Input: part model. Units: mm. Frame: model coordinates. A direction names the side the tool comes from. Give positions to 0.01 mm unless a question says otherwise; leave off trailing zeros. Order: outer loops, then holes, each group sorted by start corner. A loop starts at its lowest first (then second) coordinate and runs counter-clockwise, first axis right, second up. Notation, with made-up numbers: (-18, -30) - (31, -30) arc R8 ccw to (31, -25) - close; hole circle Ø8 at (75, 43.5). An arc over 180 degrees is marked (long way). Use a Markdown table: item, result.
from build123d import *

# Parameters (mm, degrees)
SKETCH1_W           = 200
SKETCH1_H           = 200
BOSS_EXTRUDE1_DEPTH = 6.35
CUT_EXTRUDE1_DEPTH  = 6.35
SKETCH3_R           = 1.55
CUT_EXTRUDE2_DEPTH  = 6.35


with BuildPart() as part:
    # Sketch1 → Boss-Extrude1 (new body)
    with BuildSketch(Plane.XY):
        Rectangle(SKETCH1_W, SKETCH1_H)
    extrude(amount=BOSS_EXTRUDE1_DEPTH)

    # Sketch2 → Cut-Extrude1 (cut)
    with BuildSketch(Plane.XY.offset(6.35)):
        with BuildLine():
            Line((83.65, 93.65), (-71.35, 93.65))
            ThreePointArc((-71.35, 93.65), (-78.421067812, 90.721067812), (-81.35, 83.65))
            Line((-81.35, 83.65), (-81.35, -83.65))
            ThreePointArc((-81.35, -83.65), (-78.421067812, -90.721067812), (-71.35, -93.65))
            Line((-71.35, -93.65), (83.65, -93.65))
            ThreePointArc((83.65, -93.65), (90.721067812, -90.721067812), (93.65, -83.65))
            Line((93.65, -83.65), (93.65, 83.65))
            ThreePointArc((93.65, 83.65), (90.721067812, 90.721067812), (83.65, 93.65))
        make_face()
    extrude(amount=-CUT_EXTRUDE1_DEPTH, mode=Mode.SUBTRACT)

    # Sketch3 → Cut-Extrude2 (cut)
    with BuildSketch(Plane.XY.offset(6.35)):
        with Locations((-65, -96.825)):
            Circle(SKETCH3_R)
        with Locations((65, -96.825)):
            Circle(SKETCH3_R)
        with Locations((65, 96.825)):
            Circle(SKETCH3_R)
        with Locations((-65, 96.825)):
            Circle(SKETCH3_R)
        with Locations((96.825, 32.5)):
            Circle(SKETCH3_R)
        with Locations((96.825, -32.5)):
            Circle(SKETCH3_R)
        with Locations((-96.825, 65)):
            Circle(SKETCH3_R)
        with Locations((-88.825, 65)):
            Circle(SKETCH3_R)
        with Locations((-96.825, -65)):
            Circle(SKETCH3_R)
        with Locations((-88.825, -65)):
            Circle(SKETCH3_R)
        with BuildLine():
            Line((93.65, -83.65), (93.65, 83.65))
            ThreePointArc((93.65, 83.65), (90.721067812, 90.721067812), (83.65, 93.65))
            Line((83.65, 93.65), (-71.35, 93.65))
            ThreePointArc((-71.35, 93.65), (-78.421067812, 90.721067812), (-81.35, 83.65))
            Line((-81.35, 83.65), (-81.35, -83.65))
            ThreePointArc((-81.35, -83.65), (-78.421067812, -90.721067812), (-71.35, -93.65))
            Line((-71.35, -93.65), (83.65, -93.65))
            ThreePointArc((83.65, -93.65), (90.721067812, -90.721067812), (93.65, -83.65))
        make_face()
    extrude(amount=-CUT_EXTRUDE2_DEPTH, mode=Mode.SUBTRACT)


solid = part.part
1. Section query C-C (z = 3.5). State how many separate pieces and enclosed holes the cut face has, then the cut area to 3 significant figures.
Response:
| item | result |
|---|---|
| separate pieces | 1 |
| enclosed holes | 11 |
| area | 7,230 mm^2 |
2. Section query B-B (x = -22.5). Return loops of the section in (y, z).
Response:
| item | result |
|---|---|
| outline | (-100, 0) - (-93.65, 0) - (-93.65, 6.35) - (-100, 6.35) - close; (93.65, 0) - (100, 0) - (100, 6.35) - (93.65, 6.35) - close |
3. Section query A-A (y = 9). Return loops of the section in (x, z).
Response:
| item | result |
|---|---|
| outline | (-100, 0) - (-81.35, 0) - (-81.35, 6.35) - (-100, 6.35) - close; (93.65, 0) - (100, 0) - (100, 6.35) - (93.65, 6.35) - close |
4. Material intervals for line 1 along X through (y, z) = (-65, 1.75) (3 decimals); line 2 along Y through (x, z) = (7.5, 1.5); line 3 along X through (y, z) = (22, 5.25), sorted ascending.
Response:
| item | result |
|---|---|
| line 1 | x = -100 to -98.375, -95.275 to -90.375, -87.275 to -81.35, 93.65 to 100 |
| line 2 | y = -100 to -93.65, 93.65 to 100 |
| line 3 | x = -100 to -81.35, 93.65 to 100 |
5. Pin query (flat end, axial travel): pin 1 (1.9 mm diameter, centred on x = -88.825, y = -65, fed in from +Z); pin 2 (4 mm diameter, centred on x = 65, y = -96.825, fed in from -Z). Return the tip coordinate at first contact, or that it passes through.
Response:
| item | result |
|---|---|
| pin 1 | passes through |
| pin 2 | stops at z = 0 |
6. Set-up query: faces 4 (the face through (90.8, 90.64, 3.22)), 5 (the face through (-1, 100, 3)). Return all of +Z, -Z, +X, -X, +Y, -Y with unobstructed straight access to the full face (end or side cutting, diameter ignored); none if empty.
Response:
| item | result |
|---|---|
| face 4 | +Z, -Z |
| face 5 | +Z, -Z, +X, -X, +Y |
7. Mould query, pull axis X, two halves, no side actions, for faces 1 (the face through (-100, -1, 3)), 2 (the face through (-78.34, 90.8, 3.22)), 3 (the face through (100, -1, 3)). Classes: pulls with the +X half, pulls with the -X half, needs draft (parallel to the pull), parting line crosses it, or undercut.
Response:
| item | result |
|---|---|
| face 1 | pulls with the -X half |
| face 2 | undercut |
| face 3 | pulls with the +X half |
